Here's how the part is built. I have some questions about the finished solid (model axes, mm). A direction names the side the tool comes from. Round coordinates to 2 decimals unless told otherwise and drop trailing zeros. Write each loop counter-clockwise with the first axis right and the second up, starting at its lowest first coordinate (ties: lowest second). Pieces come first, ordered by that corner, then holes. Notation, with made-up numbers: (34.5, 81.25) -> (46.5, 81.25) arc R26 ccw to (46.5, 95.25) -> close; hole circle Ø2 at (-13.75, 20.25). An arc over 180 degrees is marked (long way). Answer as CSV lines item,"result".
```python
from build123d import *

# Parameters (mm, degrees)
F1_DEPTH = 101.6
F3_DEPTH = 6.35
F4_R     = 5.55625
F5_DEPTH = 6.351
F6_R     = 5.55625
F7_DEPTH = 6.351


with BuildPart() as f1:
    # F0 (on Top) → F1 (new body)
    with BuildSketch(Plane.XY):
        Polygon((6.35, 127), (0, 127), (0, 0), (203.2, 0), (203.2, 6.35), (6.35, 6.35), align=None)
    extrude(amount=F1_DEPTH)

    # F2 (on face) → F3 (join)
    with BuildSketch(Plane(origin=(0, 0, 0), x_dir=(1, 0, 0), z_dir=(0, 0, -1))):
        Polygon((0, -127), (6.35, -127), (177.8, -6.35), (177.8, 0), (76.483584, 0), (0, -53.821781), align=None)
    extrude(amount=F3_DEPTH)

    # F4 (on face) → F5 (cut, through all)
    with BuildSketch(Plane.YZ.offset(6.35)):
        with Locations((34.925, 50.8)):
            Circle(F4_R)
        with Locations((98.425, 50.8)):
            Circle(F4_R)
    extrude(amount=-F5_DEPTH, mode=Mode.SUBTRACT)

    # F6 (on face) → F7 (cut, through all)
    with BuildSketch(Plane(origin=(0, 6.35, 0), x_dir=(-1, 0, 0), z_dir=(0, 1, 0))):
        with Locations((-152.4, 50.8)):
            Circle(F6_R)
    extrude(amount=-F7_DEPTH, mode=Mode.SUBTRACT)


solid = f1.part
```
1. On a 3-axis mill with a long thin cutter (end or side, diameter ignored), from which of +Z, -Z, +X, -X, +Y, -Y can I reach the whole of each face in a straight line? I mean faces 1 (the face through (21, 5, 0)), 2 (the face through (0, 63, 48)), 3 (the face through (203.2, 3, 50)), 4 (the face through (72, 52, 0)), 5 (the face through (177.8, 3, -3)). Say none if no direction works.
Numbers:
face 1,"-Z, -X, -Y"
face 2,"+Z, -Z, -X, +Y, -Y"
face 3,"+Z, -Z, +X, +Y, -Y"
face 4,"+Z, +X, +Y"
face 5,"-Z, +X, +Y, -Y"
2. For pin 1 Ø4 at (x, y) = (60.5, 56.5) entering from +Z; pin 2 Ø10 at (y, z) = (71.5, 81) entering from +X; pin 3 Ø4 at (x, z) = (42, 42.5) entering from +Y, each with a flat end and sliding along its axis, tell me the tip position at first contact or that it passes through.
Numbers:
pin 1,"stops at z = 0"
pin 2,"stops at x = 6.35"
pin 3,"stops at y = 6.35"
3. Suppose I cut it at D-D on y = 70. Please give me the cut outline in (x, z).
Numbers:
outline,"(0, -6.35) -> (87.35, -6.35) -> (87.35, 0) -> (6.35, 0) -> (6.35, 101.6) -> (0, 101.6) -> close"
4. If I drill on line 1 (Y direction, x = 170, z = 88.5); line 2 (Z direction, x = 152.4, y = 1.75), over which ranges is the centre line in solid material (lowest first)?
Numbers:
line 1,"y = 0 to 6.35"
line 2,"z = -6.35 to 45.24, 56.36 to 101.6"
5. Suppose I cut it at C-C on y = 46. Please give me the cut outline in (x, z), and give its area (3 significant figures).
Numbers:
outline,"(0, 0) -> (6.35, 0) -> (6.35, 101.6) -> (0, 101.6) -> close; (11.12, -6.35) -> (121.46, -6.35) -> (121.46, 0) -> (11.12, 0) -> close"
area,"1,350 mm^2"
6. Suppose I cut it at B-B on x = 153.5. Please give me the cut outline in (y, z), and give its area (3 significant figures).
Numbers:
outline,"(0, -6.35) -> (23.45, -6.35) -> (23.45, 0) -> (6.35, 0) -> (6.35, 45.35) -> (0, 45.35) -> close; (0, 56.25) -> (6.35, 56.25) -> (6.35, 101.6) -> (0, 101.6) -> close"
area,"725 mm^2"
7. Suppose I cut it at A-A on z = 50.8. Please give me the cut outline in (x, y), and give its area (3 significant figures).
Numbers:
outline,"(0, 0) -> (146.84, 0) -> (146.84, 6.35) -> (6.35, 6.35) -> (6.35, 29.37) -> (0, 29.37) -> close; (0, 40.48) -> (6.35, 40.48) -> (6.35, 92.87) -> (0, 92.87) -> close; (0, 103.98) -> (6.35, 103.98) -> (6.35, 127) -> (0, 127) -> close; (157.96, 0) -> (203.2, 0) -> (203.2, 6.35) -> (157.96, 6.35) -> close"
area,"1,840 mm^2"
8. If we mould it in two halves opening along Z, with no side actions, what happens to faces 6 (the face through (3, 127, 48)), 7 (the face through (3.219, 103.725, 52.469)), 8 (the face through (56, 3, 101.6))? For each: released by +Z, released by -Z, zero draft, split by the parting line, or undercut.
Numbers:
face 6,"zero draft"
face 7,"undercut"
face 8,"released by +Z"
